The listing builds one solid part. Answer for the finished solid, in the listing's coordinates (mm). Round coordinates to 2 decimals unless told otherwise and drop trailing zeros. Write each loop counter-clockwise with the first axis right and the second up, starting at its lowest first coordinate (ties: lowest second). Pieces come first, ordered by that corner, then holes.
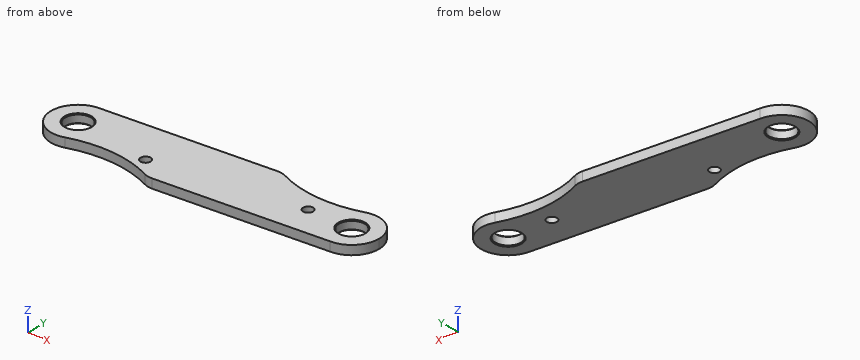
from build123d import *

# Parameters (mm, degrees)
CROQUIS1_R              = 16.5
SALIENTE_EXTRUIR1_DEPTH = 11.7
SALIENTE_EXTRUIR6_START = -11.7
CROQUIS9_R              = 16.5
SALIENTE_EXTRUIR6_DEPTH = 11.7
SALIENTE_EXTRUIR5_START = -11.7
CROQUIS8_R              = 35
CROQUIS8_R_2            = 16.5
CROQUIS8_R_3            = 22.5
SALIENTE_EXTRUIR5_DEPTH = 11.7
CHAFL_N1_SIZE           = 1
CORTAR_EXTRUIR7_REACH   = 217.086
CROQUIS19_R             = 6.5


with BuildPart() as part:
    # Croquis1 → Saliente-Extruir1 (new body)
    with BuildSketch(Plane.XY):
        with BuildLine():
            Line((-197.5, 25), (197.5, 25))
            ThreePointArc((197.5, 25), (203.120875688, 0), (197.5, -25))
            Line((197.5, -25), (-197.5, -25))
            ThreePointArc((-197.5, -25), (-203.120875688, 0), (-197.5, 25))
        make_face()
        with Locations((-175, 0)):
            Circle(CROQUIS1_R, mode=Mode.SUBTRACT)
        with Locations((175, 0)):
            Circle(CROQUIS1_R, mode=Mode.SUBTRACT)
    extrude(amount=SALIENTE_EXTRUIR1_DEPTH)

    # Croquis9 → Saliente-Extruir6 (add)
    # profile 1 of 17: a face of its own
    with BuildSketch(Plane.XY.offset(11.7).offset(SALIENTE_EXTRUIR6_START)):
        with BuildLine():
            ThreePointArc((-140, 0), (-142.732978058, 13.558735008), (-150.505102572, 25))
            Line((-150.505102572, 25), (-197.5, 25))
            ThreePointArc((-197.5, 25), (-203.120875688, 0), (-197.5, -25))
            Line((-197.5, -25), (-150.505102572, -25))
            ThreePointArc((-150.505102572, -25), (-142.732978058, -13.558735008), (-140, 0))
        make_face()
        with Locations((-175, 0)):
            Circle(CROQUIS9_R, mode=Mode.SUBTRACT)
    # profile 2 of 17: a face of its own
    with BuildSketch(Plane.XY.offset(11.7).offset(SALIENTE_EXTRUIR6_START)):
        with BuildLine():
            ThreePointArc((-150.505102572, 25), (-161.771243445, 32.403703492), (-175, 35))
            ThreePointArc((-175, 35), (-209.624362587, -5.114050788), (-164.881671498, -33.505513402))
            ThreePointArc((-164.881671498, -33.505513402), (-157.178530031, -30.123001313), (-150.505102572, -25))
            Line((-150.505102572, -25), (-197.5, -25))
            ThreePointArc((-197.5, -25), (-203.120875688, 0), (-197.5, 25))
            Line((-197.5, 25), (-150.505102572, 25))
        make_face()
    # profile 3 of 17: a face of its own
    with BuildSketch(Plane.XY.offset(11.7).offset(SALIENTE_EXTRUIR6_START)):
        with BuildLine():
            Line((43.975947947, 44.976683861), (-175, 35))
            ThreePointArc((-175, 35), (-161.771243445, 32.403703492), (-150.505102572, 25))
            Line((-150.505102572, 25), (22.639320225, 25))
            ThreePointArc((22.639320225, 25), (29.62214595, 38.92472541), (43.975947947, 44.976683861))
        make_face()
    # profile 4 of 17: a face of its own
    with BuildSketch(Plane.XY.offset(11.7).offset(SALIENTE_EXTRUIR6_START)):
        with BuildLine():
            Line((22.639320225, 25), (-150.505102572, 25))
            ThreePointArc((-150.505102572, 25), (-142.732978058, 13.558735008), (-140, 0))
            ThreePointArc((-140, 0), (-142.732978058, -13.558735008), (-150.505102572, -25))
            Line((-150.505102572, -25), (-67.360679775, -25))
            ThreePointArc((-67.360679775, -25), (-46.251939508, -0.034857057), (-22.5, -22.5))
            ThreePointArc((-22.5, -22.5), (-22.534857057, -23.751939508), (-22.639320225, -25))
            Line((-22.639320225, -25), (150.505102572, -25))
            ThreePointArc((150.505102572, -25), (140, 0), (150.505102572, 25))
            Line((150.505102572, 25), (67.360679775, 25))
            ThreePointArc((67.360679775, 25), (67.465142943, 23.751939508), (67.5, 22.5))
            ThreePointArc((67.5, 22.5), (43.748060492, 0.034857057), (22.639320225, 25))
        make_face()
    # profile 5 of 17: a face of its own
    with BuildSketch(Plane.XY.offset(11.7).offset(SALIENTE_EXTRUIR6_START)):
        with BuildLine():
            ThreePointArc((-150.505102572, -25), (-157.178530031, -30.123001313), (-164.881671498, -33.505513402))
            ThreePointArc((-164.881671498, -33.505513402), (-109.058760851, -27.618859086), (-54.980531281, -42.665291849))
            ThreePointArc((-54.980531281, -42.665291849), (-63.425637497, -35.413012152), (-67.360679775, -25))
            Line((-67.360679775, -25), (-150.505102572, -25))
        make_face()
    # profile 6 of 17: a face of its own
    with BuildSketch(Plane.XY.offset(11.7).offset(SALIENTE_EXTRUIR6_START)):
        with BuildLine():
            ThreePointArc((-67.360679775, -25), (-63.425637497, -35.413012152), (-54.980531281, -42.665291849))
            ThreePointArc((-54.980531281, -42.665291849), (-49.624960897, -44.519530801), (-43.975947947, -44.976683861))
            ThreePointArc((-43.975947947, -44.976683861), (-29.62214595, -38.92472541), (-22.639320225, -25))
            Line((-22.639320225, -25), (-67.360679775, -25))
        make_face()
    # profile 7 of 17: a face of its own
    with BuildSketch(Plane.XY.offset(11.7).offset(SALIENTE_EXTRUIR6_START)):
        with BuildLine():
            ThreePointArc((-22.5, -22.5), (-46.251939508, -0.034857057), (-67.360679775, -25))
            Line((-67.360679775, -25), (-22.639320225, -25))
            ThreePointArc((-22.639320225, -25), (-22.534857057, -23.751939508), (-22.5, -22.5))
        make_face()
    # profile 8 of 17: a face of its own
    with BuildSketch(Plane.XY.offset(11.7).offset(SALIENTE_EXTRUIR6_START)):
        with BuildLine():
            ThreePointArc((-67.360679775, -25), (-63.425637497, -35.413012152), (-54.980531281, -42.665291849))
            ThreePointArc((-54.980531281, -42.665291849), (-49.624960897, -44.519530801), (-43.975947947, -44.976683861))
            ThreePointArc((-43.975947947, -44.976683861), (-29.62214595, -38.92472541), (-22.639320225, -25))
            Line((-22.639320225, -25), (-67.360679775, -25))
        make_face()
    # profile 9 of 17: a face of its own
    with BuildSketch(Plane.XY.offset(11.7).offset(SALIENTE_EXTRUIR6_START)):
        with BuildLine():
            ThreePointArc((-22.5, -22.5), (-46.251939508, -0.034857057), (-67.360679775, -25))
            Line((-67.360679775, -25), (-22.639320225, -25))
            ThreePointArc((-22.639320225, -25), (-22.534857057, -23.751939508), (-22.5, -22.5))
        make_face()
    # profile 10 of 17: a face of its own
    with BuildSketch(Plane.XY.offset(11.7).offset(SALIENTE_EXTRUIR6_START)):
        with BuildLine():
            ThreePointArc((54.980531281, 42.665291849), (49.624960897, 44.519530801), (43.975947947, 44.976683861))
            ThreePointArc((43.975947947, 44.976683861), (29.62214595, 38.92472541), (22.639320225, 25))
            Line((22.639320225, 25), (67.360679775, 25))
            ThreePointArc((67.360679775, 25), (63.425637497, 35.413012152), (54.980531281, 42.665291849))
        make_face()
    # profile 11 of 17: a face of its own
    with BuildSketch(Plane.XY.offset(11.7).offset(SALIENTE_EXTRUIR6_START)):
        with BuildLine():
            Line((67.360679775, 25), (22.639320225, 25))
            ThreePointArc((22.639320225, 25), (43.748060492, 0.034857057), (67.5, 22.5))
            ThreePointArc((67.5, 22.5), (67.465142943, 23.751939508), (67.360679775, 25))
        make_face()
    # profile 12 of 17: a face of its own
    with BuildSketch(Plane.XY.offset(11.7).offset(SALIENTE_EXTRUIR6_START)):
        with BuildLine():
            ThreePointArc((54.980531281, 42.665291849), (49.624960897, 44.519530801), (43.975947947, 44.976683861))
            ThreePointArc((43.975947947, 44.976683861), (29.62214595, 38.92472541), (22.639320225, 25))
            Line((22.639320225, 25), (67.360679775, 25))
            ThreePointArc((67.360679775, 25), (63.425637497, 35.413012152), (54.980531281, 42.665291849))
        make_face()
    # profile 13 of 17: a face of its own
    with BuildSketch(Plane.XY.offset(11.7).offset(SALIENTE_EXTRUIR6_START)):
        with BuildLine():
            Line((67.360679775, 25), (22.639320225, 25))
            ThreePointArc((22.639320225, 25), (43.748060492, 0.034857057), (67.5, 22.5))
            ThreePointArc((67.5, 22.5), (67.465142943, 23.751939508), (67.360679775, 25))
        make_face()
    # profile 14 of 17: a face of its own
    with BuildSketch(Plane.XY.offset(11.7).offset(SALIENTE_EXTRUIR6_START)):
        with BuildLine():
            ThreePointArc((164.881671498, 33.505513402), (109.058760851, 27.618859086), (54.980531281, 42.665291849))
            ThreePointArc((54.980531281, 42.665291849), (63.425637497, 35.413012152), (67.360679775, 25))
            Line((67.360679775, 25), (150.505102572, 25))
            ThreePointArc((150.505102572, 25), (157.178530031, 30.123001313), (164.881671498, 33.505513402))
        make_face()
    # profile 15 of 17: a face of its own
    with BuildSketch(Plane.XY.offset(11.7).offset(SALIENTE_EXTRUIR6_START)):
        with BuildLine():
            ThreePointArc((-22.639320225, -25), (-29.62214595, -38.92472541), (-43.975947947, -44.976683861))
            Line((-43.975947947, -44.976683861), (175, -35))
            ThreePointArc((175, -35), (161.771243445, -32.403703492), (150.505102572, -25))
            Line((150.505102572, -25), (-22.639320225, -25))
        make_face()
    # profile 16 of 17: a face of its own
    with BuildSketch(Plane.XY.offset(11.7).offset(SALIENTE_EXTRUIR6_START)):
        with BuildLine():
            ThreePointArc((210, 0), (195.866941588, 28.099301571), (164.881671498, 33.505513402))
            ThreePointArc((164.881671498, 33.505513402), (157.178530031, 30.123001313), (150.505102572, 25))
            Line((150.505102572, 25), (197.5, 25))
            ThreePointArc((197.5, 25), (203.120875688, 0), (197.5, -25))
            Line((197.5, -25), (150.505102572, -25))
            ThreePointArc((150.505102572, -25), (161.771243445, -32.403703492), (175, -35))
            ThreePointArc((175, -35), (199.748737342, -24.748737342), (210, 0))
        make_face()
    # profile 17 of 17: a face of its own
    with BuildSketch(Plane.XY.offset(11.7).offset(SALIENTE_EXTRUIR6_START)):
        with BuildLine():
            Line((197.5, 25), (150.505102572, 25))
            ThreePointArc((150.505102572, 25), (140, 0), (150.505102572, -25))
            Line((150.505102572, -25), (197.5, -25))
            ThreePointArc((197.5, -25), (203.120875688, 0), (197.5, 25))
        make_face()
        with Locations((175, 0)):
            Circle(CROQUIS9_R, mode=Mode.SUBTRACT)
    extrude(amount=SALIENTE_EXTRUIR6_DEPTH)

    # Croquis8 → Saliente-Extruir5 (add)
    # profile 1 of 4: a face of its own
    with BuildSketch(Plane.XY.offset(11.7).offset(SALIENTE_EXTRUIR5_START)):
        with Locations((-175, 0)):
            Circle(CROQUIS8_R)
        with Locations((-175, 0)):
            Circle(CROQUIS8_R_2, mode=Mode.SUBTRACT)
    # profile 2 of 4: a face of its own
    with BuildSketch(Plane.XY.offset(11.7).offset(SALIENTE_EXTRUIR5_START)):
        with Locations((175, 0)):
            Circle(CROQUIS8_R)
        with Locations((175, 0)):
            Circle(CROQUIS8_R_2, mode=Mode.SUBTRACT)
    # profile 3 of 4: a face of its own
    with BuildSketch(Plane.XY.offset(11.7).offset(SALIENTE_EXTRUIR5_START)):
        with Locations((45, 22.5)):
            Circle(CROQUIS8_R_3)
    # profile 4 of 4: a face of its own
    with BuildSketch(Plane.XY.offset(11.7).offset(SALIENTE_EXTRUIR5_START)):
        with Locations((-45, -22.5)):
            Circle(CROQUIS8_R_3)
    extrude(amount=SALIENTE_EXTRUIR5_DEPTH)

    # Chaflán1
    chafl_n1_edges = [part.edges().sort_by_distance(p)[0] for p in [
        (-191.5, 0, 0),
        (-191.5, 0, 11.7),
        (158.5, 0, 0),
        (158.5, 0, 11.7),
    ]]
    chamfer(chafl_n1_edges, length=CHAFL_N1_SIZE)

    # Croquis19 → Cortar-Extruir7 (cut, up to next)
    with BuildSketch(Plane(origin=(0, 0, 0), x_dir=(-1, 0, 0), z_dir=(0, 0, -1)), mode=Mode.PRIVATE) as cortar_extruir7_sk1:
        with Locations((73.534579942, -18.901548417)):
            Circle(CROQUIS19_R)
    cortar_extruir7_tool1 = extrude(cortar_extruir7_sk1.sketch, amount=-CORTAR_EXTRUIR7_REACH, mode=Mode.PRIVATE) & part.part
    # Croquis19 → Cortar-Extruir7 (cut, up to next)
    with BuildSketch(Plane(origin=(0, 0, 0), x_dir=(-1, 0, 0), z_dir=(0, 0, -1)), mode=Mode.PRIVATE) as cortar_extruir7_sk2:
        with Locations((-117.200528877, 2.301431648)):
            Circle(CROQUIS19_R)
    cortar_extruir7_tool2 = extrude(cortar_extruir7_sk2.sketch, amount=-CORTAR_EXTRUIR7_REACH, mode=Mode.PRIVATE) & part.part
    add(cortar_extruir7_tool1.solids().sort_by_distance((-73.53458, -18.901548, 0))[0], mode=Mode.SUBTRACT)
    add(cortar_extruir7_tool2.solids().sort_by_distance((117.200529, 2.301432, 0))[0], mode=Mode.SUBTRACT)


solid = part.part
1. Section B-B on x = -86.5 is taken. Determine the outline of the cut face in (y, z), plus the area to 3 significant figures.
Geometry says:
outline: (-31.25, 0) - (39.03, 0) - (39.03, 11.7) - (-31.25, 11.7) - close
area: 822 mm2
2. Given pin 1 (5 mm diameter, centred on x = -154, z = 8.5, fed in from +Y); pin 2 (1 mm diameter, centred on y = -26.5, z = 2, fed in from +X); pin 3 (2 mm diameter, centred on y = 7.5, z = 6.5, fed in from -X), each flat-ended and moving along its own axis, determine where each tip first touches the part or whether it passes through.
Geometry says:
pin 1: stops at y = 36.07
pin 2: stops at x = 198.43
pin 3: stops at x = -209.39
3. Section A-A on z = 3.75 is taken. Determine the outline of the cut face in (x, y), plus the area to 3 significant figures.
Geometry says:
outline: (-175, 35) arc R35 ccw (long way) to (-164.88, -33.51) arc R150 cw to (-54.98, -42.67) arc R22.5 ccw to (-43.98, -44.98) - (175, -35) arc R35 ccw (long way) to (164.88, 33.51) arc R150 cw to (54.98, 42.67) arc R22.5 ccw to (43.98, 44.98) - close; hole circle Ø33 at (-175, 0); hole circle Ø13 at (-73.53, -18.9); hole circle Ø13 at (117.2, 2.3); hole circle Ø33 at (175, 0)
area: 27,900 mm2
4. Straight lines are drawn through the part: line 1 along X through (y, z) = (9.5, 6); line 2 along X through (y, z) = (10, 3); line 3 along X through (y, z) = (6, 5). For each, find the intervals that lie inside material, in ascending order.
Geometry says:
line 1: x = -208.69 to -188.49, -161.51 to 161.51, 188.49 to 208.69
line 2: x = -208.54 to -188.12, -161.88 to 161.88, 188.12 to 208.54
line 3: x = -209.48 to -190.37, -159.63 to 111.86, 122.55 to 159.63, 190.37 to 209.48
